Job drawing, mm, ordinate dimensions from the low corner. One solid piece. A direction names the side the tool comes from. Round coordinates to 2 decimals unless told otherwise and drop trailing zeros. Loops run counter-clockwise (first coordinate to the right, second up) from the corner with the lowest first, then second, coordinate; pieces in that order, holes last. Notation, with made-up numbers: M 52,58.25 L 78,58.25 A35 cw 78,90.25 Z; hole C 14.25,13.5 d2. An arc over 180 degrees is marked long. Use one line per item in the form item = value.
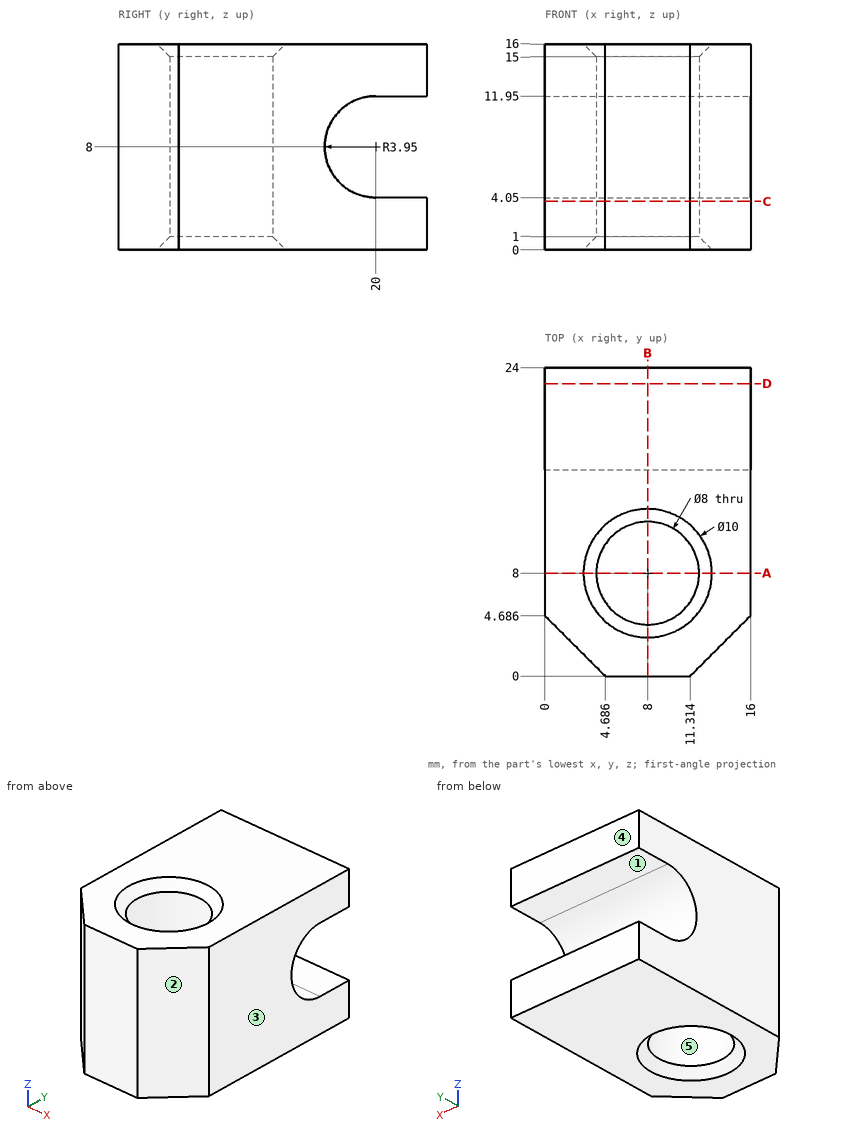
1. Cut at A-A on y = 8. Write the cut outline in (x, z).
Completed:
outline = M 0,0 L 3,0 L 4,1 L 4,15 L 3,16 L 0,16 Z; M 12,1 L 13,0 L 16,0 L 16,16 L 13,16 L 12,15 Z
2. Cut at C-C on z = 3.75. Write the cut outline in (x, y).
Completed:
outline = M 0,4.69 L 4.69,0 L 11.31,0 L 16,4.69 L 16,24 L 0,24 Z; hole C 8,8 d8
3. Probe line 1 along X through (y, z) = (10.25, 5); line 2 along Z through (x, y) = (9, 22). List the from-to ranges inside material, lowest first. Write a range as from..to.
Completed:
line_1 = 0..4.69, 11.31..16
line_2 = 0..4.05, 11.95..16
4. Drop a flat-ended pin along its axis: P1, Ø1.5, axis at x = 3, z = 14.5, coming from the -Y side. Give the stop position or say it passes through.
Completed:
P1 = 0.94
5. Tool access for the marked faces 1 and 2: list every direction of +Z, -Z, +X, -X, +Y, -Y with a clear straight run to the whole face (end or side of a thin tool).
Completed:
face_1 = +X, -X, +Y
face_2 = +Z, -Z, +X, -Y
6. Cut at B-B on x = 8. Write the cut outline in (y, z).
Completed:
outline = M 0,0 L 3,0 L 4,1 L 4,15 L 3,16 L 0,16 Z; M 12,1 L 13,0 L 24,0 L 24,4.05 L 20,4.05 A3.95 cw 20,11.95 L 24,11.95 L 24,16 L 13,16 L 12,15 Z
7. Pull direction X, two halves, no side cores. Call the marked faces 3, 4 and 5: +X half, -X half, draft (parallel to the pull), parting line (faces both ways), or undercut.
Completed:
face_3 = +X half
face_4 = draft
face_5 = undercut
8. Cut at D-D on y = 22.75. Write the cut outline in (x, z), and give its area (3 significant figures).
Completed:
outline = M 0,0 L 16,0 L 16,4.05 L 0,4.05 Z; M 0,11.95 L 16,11.95 L 16,16 L 0,16 Z
area = 130 mm2
